Check sheet for the modelled part. Datum: model origin and axes. Units: mm. A direction names the side the tool comes from. Round coordinates to 2 decimals unless told otherwise and drop trailing zeros. Write each loop counter-clockwise with the first axis right and the second up, starting at its lowest first coordinate (ties: lowest second). Pieces come first, ordered by that corner, then holes. Notation, with made-up numbers: (74.25, 19.5) - (132.25, 19.5) arc R24 ccw to (132.25, 44.5) - close; hole circle Ø1 at (57.25, 14.5). An arc over 180 degrees is marked (long way). Answer as a JSON object with one key per item and string values. Group by question number.
Item 1: Sectioned sample at C-C on x = 0. Record the boundary of the cut face in (y, z).
Item 2: Sectioned sample at B-B on y = -18. Record the boundary of the cut face in (x, z), plus the area to 3 significant figures.
Item 3: Gauge pin test, flat ends, axial feed: P1, Ø1, axis at y = 9.5, z = -7.5, coming from the -X side; P2, Ø5, axis at y = -0.5, z = 7.5, coming from the +X side; P3, Ø10, axis at x = 0.5, z = 22.5, coming from the +Y side; P4, Ø4, axis at y = -3.5, z = 19, coming from the -X side. Record the tip position at first contact, or that the pin passes through.
Item 4: Sectioned sample at A-A on x = 6.25. Record the boundary of the cut face in (y, z).
Item 5: Set-up check for faces 1 (the cylindrical face through (-2.753, 17.621, 0.088)), 2 (the cylindrical face through (-2.75, -12.52, -12.4)): record each of +Z, -Z, +X, -X, +Y, -Y from which the full face is reachable in a straight line by a thin tool's end or side.
Item 6: Thickness scan on line 1 (Y direction, x = 3.5, z = 8) (3 decimals); line 2 (Z direction, x = -8.5, y = -11); line 3 (X direction, y = 16.5, z = 17). Record the ranges inside material, lowest first.
```python
from build123d import *

# Parameters (mm, degrees)
F5_R     = 12.7
F6_DEPTH = 25.4


# Not quite as in the source:
# - a feature of the source that left no trace in its solid (it failed there, or was rolled back) is left out
# - a pattern or mirror of a feature is missing from the dataset's text; its kind, count and spacing are read off the source's solid


with BuildPart() as f4:
    # F3 (on Right) → F4 (revolve)
    with BuildSketch(Plane.YZ):
        with BuildLine():
            Line((0, -12.7), (0, 12.7))
            ThreePointArc((0, 12.7), (-12.7, 0), (0, -12.7))
        make_face()
    revolve(axis=Axis((0, 0, -2.0618988201), (0, 0, -1)))

    # F5 (on Front) → F6 (join)
    with BuildSketch(Plane.XZ):
        Circle(F5_R)
    f6 = extrude(amount=F6_DEPTH)

    # F6_copies: F6 across plane
    add(f6.mirror(Plane(origin=(0, 0, 0), x_dir=(0, -0.3826834324, 0.9238795325), z_dir=(0, 0.9238795325, 0.3826834324))))


solid = f4.part
```
Completed:
{
 "1": {"outline": "(-25.4, -12.7) - (0, -12.7) arc R12.7 ccw to (8.98, -8.98) - (26.94, 8.98) - (8.98, 26.94) - (-5.26, 12.7) - (-25.4, 12.7) - close"},
 "2": {"outline": "circle Ø25.4 at (0, 0)", "area": "507 mm²"},
 "3": {"P1": "x = -5.34", "P2": "x = 12.3", "P3": "y = 18.42", "P4": "through"},
 "4": {"outline": "(-25.4, -11.06) - (0, -11.06) arc R11.06 ccw to (7.82, -7.82) - (25.78, 10.14) - (10.14, 25.78) - (-4.58, 11.06) - (-25.4, 11.06) - close"},
 "5": {"face 1": "none", "face 2": "-Y"},
 "6": {"line 1": "-25.4 to 25.265", "line 2": "-9.44 to 9.44", "line 3": "-12.7 to 12.7"}
}
